```python
from build123d import *

# Parameters (mm, degrees)
SKETCH1_W           = 75
SKETCH1_H           = 75
SKETCH1_R           = 2.75
SKETCH1_R_2         = 16
BOSS_EXTRUDE1_DEPTH = 6
BOSS_EXTRUDE2_DEPTH = 75
SKETCH3_R           = 21.05
CUT_EXTRUDE1_DEPTH  = 6
SKETCH4_R           = 21.05
SKETCH4_R_2         = 19.05
BOSS_EXTRUDE3_DEPTH = 2
SKETCH5_R           = 3.25
CUT_EXTRUDE2_DEPTH  = 97.785892457
CUT_EXTRUDE3_DEPTH  = 6
SKETCH7_R           = 1.25
BOSS_EXTRUDE4_DEPTH = 10
SKETCH11_W          = 6.5
SKETCH11_H          = 26
CUT_EXTRUDE7_DEPTH  = 10


with BuildPart() as part:
    # Sketch1 → Boss-Extrude1 (new body)
    with BuildSketch(Plane.XY):
        Rectangle(SKETCH1_W, SKETCH1_H)
        with Locations((21, 21)):
            Circle(SKETCH1_R, mode=Mode.SUBTRACT)
        with Locations((21, -21)):
            Circle(SKETCH1_R, mode=Mode.SUBTRACT)
        with Locations((-21, -21)):
            Circle(SKETCH1_R, mode=Mode.SUBTRACT)
        with Locations((-21, 21)):
            Circle(SKETCH1_R, mode=Mode.SUBTRACT)
        Circle(SKETCH1_R_2, mode=Mode.SUBTRACT)
    extrude(amount=BOSS_EXTRUDE1_DEPTH)

    # Sketch2 → Boss-Extrude2 (add)
    with BuildSketch(Plane.ZY.offset(37.5)):
        Polygon((0, 37.5), (-50, 37.5), (-50, 69.464084092), (-55, 69.464084092), (-55, 32.5), (-36.09839393, 32.5), (-36.09839393, -32.5), (-55, -32.5), (-55, -69.464084092), (-50, -69.464084092), (-50, -37.5), (0, -37.5), (0, -32.5), (-30.09839393, -32.5), (-30.09839393, 32.5), (0, 32.5), align=None)
    extrude(amount=-BOSS_EXTRUDE2_DEPTH)

    # Sketch3 → Cut-Extrude1 (cut)
    with BuildSketch(Plane(origin=(0, 0, -36.09839393), x_dir=(-1, 0, 0), z_dir=(0, 0, -1))):
        Circle(SKETCH3_R)
    extrude(amount=-CUT_EXTRUDE1_DEPTH, mode=Mode.SUBTRACT)

    # Sketch4 → Boss-Extrude3 (add)
    with BuildSketch(Plane(origin=(0, 0, -36.09839393), x_dir=(-1, 0, 0), z_dir=(0, 0, -1))):
        Circle(SKETCH4_R)
        Circle(SKETCH4_R_2, mode=Mode.SUBTRACT)
    extrude(amount=-BOSS_EXTRUDE3_DEPTH)

    # Sketch5 → Cut-Extrude2 (cut, through all)
    with BuildSketch(Plane.XY.offset(-50)):
        with Locations((30, -60)):
            Circle(SKETCH5_R)
        with Locations((-30, -60)):
            Circle(SKETCH5_R)
    cut_extrude2 = extrude(amount=-CUT_EXTRUDE2_DEPTH, mode=Mode.SUBTRACT)

    # Mirror1: Cut-Extrude2 across plane
    add(cut_extrude2.mirror(Plane.ZX), mode=Mode.SUBTRACT)

    # Sketch6 → Cut-Extrude3 (cut)
    with BuildSketch(Plane(origin=(0, 0, -36.09839393), x_dir=(-1, 0, 0), z_dir=(0, 0, -1))):
        with BuildLine():
            Line((26, 23.5), (26, 18.5))
            ThreePointArc((26, 18.5), (21, 13.5), (16, 18.5))
            Line((16, 18.5), (16, 23.5))
            ThreePointArc((16, 23.5), (21, 28.5), (26, 23.5))
        make_face()
        with BuildLine():
            Line((16, -23.5), (16, -18.5))
            ThreePointArc((16, -18.5), (21, -13.5), (26, -18.5))
            Line((26, -18.5), (26, -23.5))
            ThreePointArc((26, -23.5), (21, -28.5), (16, -23.5))
        make_face()
        with BuildLine():
            Line((-16, -23.5), (-16, -18.5))
            ThreePointArc((-16, -18.5), (-21, -13.5), (-26, -18.5))
            Line((-26, -18.5), (-26, -23.5))
            ThreePointArc((-26, -23.5), (-21, -28.5), (-16, -23.5))
        make_face()
        with BuildLine():
            Line((-26, 23.5), (-26, 18.5))
            ThreePointArc((-26, 18.5), (-21, 13.5), (-16, 18.5))
            Line((-16, 18.5), (-16, 23.5))
            ThreePointArc((-16, 23.5), (-21, 28.5), (-26, 23.5))
        make_face()
    extrude(amount=-CUT_EXTRUDE3_DEPTH, mode=Mode.SUBTRACT)

    # Sketch7 → Boss-Extrude4 (add)
    # profile 1 of 2: a face of its own
    with BuildSketch(Plane(origin=(0, 0, -36.09839393), x_dir=(-1, 0, 0), z_dir=(0, 0, -1))):
        Polygon((-26, -3), (-21, -3), (-21, -13), (-37.5, -13), (-37.5, -10), (-26, -10), align=None)
        with Locations(Location((-23.5, -5, 0), (0, 0, 180))):
            Circle(SKETCH7_R, mode=Mode.SUBTRACT)
    # profile 2 of 2: a face of its own
    with BuildSketch(Plane(origin=(0, 0, -36.09839393), x_dir=(-1, 0, 0), z_dir=(0, 0, -1))):
        Polygon((-21, 13), (-37.5, 13), (-37.5, 10), (-26, 10), (-26, 3), (-21, 3), align=None)
        with Locations((-23.5, 5)):
            Circle(SKETCH7_R, mode=Mode.SUBTRACT)
    extrude(amount=BOSS_EXTRUDE4_DEPTH)

    # Sketch11 → Cut-Extrude7 (cut)
    with BuildSketch(Plane.ZY.offset(-21)):
        with Locations((-39.34839393, 0)):
            Rectangle(SKETCH11_W, SKETCH11_H)
    extrude(amount=-CUT_EXTRUDE7_DEPTH, mode=Mode.SUBTRACT)


solid = part.part
```
Geometry: final body of the model. Coordinates: model frame, mm. A direction names the side the tool comes from. Round coordinates to 2 decimals unless told otherwise and drop trailing zeros. Order: outer loops, then holes, each group sorted by start corner. A loop starts at its lowest first (then second) coordinate and runs counter-clockwise, first axis right, second up. Notation, with made-up numbers: (-28.75, 60.25) -> (8.25, 60.25) arc R27 ccw to (8.25, 86.25) -> close; hole circle Ø3 at (79, 3). An arc over 180 degrees is marked (long way). Write each question's results on one line, items separated by ' | '.
Q1. Pull-direction query (Y, two-part tool) for faces 1 (the face through (18.253, 21.121, 2.958)), 2 (the face through (-1, -37.5, -22)), 3 (the face through (-1, -54, -50)); classes: released by +Y, released by -Y, zero draft, split by the parting line, or undercut.
Response values:
face 1: undercut | face 2: released by -Y | face 3: zero draft
Q2. Section query C-C (y = 60). Output: boundary loops of the cut face in (x, z).
Response values:
outline: (-37.5, -55) -> (-33.25, -55) -> (-33.25, -50) -> (-37.5, -50) -> close; (-26.75, -55) -> (26.75, -55) -> (26.75, -50) -> (-26.75, -50) -> close; (33.25, -55) -> (37.5, -55) -> (37.5, -50) -> (33.25, -50) -> close
Q3. Section query D-D (y = -30.5). Output: boundary loops of the cut face in (x, z), and give its area (3 significant figures).
Response values:
outline: (-37.5, -36.1) -> (37.5, -36.1) -> (37.5, -30.1) -> (-37.5, -30.1) -> close; (-37.5, 0) -> (37.5, 0) -> (37.5, 6) -> (-37.5, 6) -> close | area: 900 mm²
Q4. Section query B-B (z = -40). Output: boundary loops of the cut face in (x, y), and give its area (3 significant figures).
Response values:
outline: (-37.5, -37.5) -> (37.5, -37.5) -> (37.5, -32.5) -> (-37.5, -32.5) -> close; (-37.5, 32.5) -> (37.5, 32.5) -> (37.5, 37.5) -> (-37.5, 37.5) -> close; (31, -13) -> (37.5, -13) -> (37.5, -10) -> (31, -10) -> close; (31, 10) -> (37.5, 10) -> (37.5, 13) -> (31, 13) -> close | area: 789 mm²
Q5. Access query for faces 4 (the face through (-1, 53, -50)), 5 (the face through (-21.1, -28.5, -33.1)), 6 (the face through (31, -11, -39)), 7 (the face through (24, -3, -44)). Directions: +Z, -Z, +X, -X, +Y, -Y. A direction counts if a zero-diameter tool reaches every point of the face in a straight line with its end or side. Return the directions, or none.
Response values:
face 4: +Z, +X, -X, +Y | face 5: -Z | face 6: -X | face 7: -Z, +X, -X
Q6. Pin query (flat end, axial travel): pin 1 Ø1.8 at (x, z) = (22.5, -45) entering from +Y; pin 2 Ø11 at (x, y) = (26, 9.5) entering from -Z; pin 3 Ø1.5 at (x, z) = (-0.5, -38.5) entering from -Y; pin 4 Ø5 at (x, y) = (21, 21) entering from -Z. Return the tip coordinate at first contact, or that it passes through.
Response values:
pin 1: y = 37.5 | pin 2: z = -46.1 | pin 3: y = -37.5 | pin 4: through
Q7. Ray query, line 1 along X through (y, z) = (60, -52.7); line 2 along Y through (x, z) = (30, -53); line 3 along Y through (x, z) = (-6.5, -13). Return the intervals inside material, ascending.
Response values:
line 1: -37.5 to -33.25, -26.75 to 26.75, 33.25 to 37.5 | line 2: -69.46 to -63.25, -56.75 to -32.5, 32.5 to 56.75, 63.25 to 69.46 | line 3: -37.5 to -32.5, 32.5 to 37.5
Q8. Section query A-A (x = -30). Output: boundary loops of the cut face in (y, z), and give its area (3 significant figures).
Response values:
outline: (-69.46, -55) -> (-63.25, -55) -> (-63.25, -50) -> (-69.46, -50) -> close; (-56.75, -55) -> (-32.5, -55) -> (-32.5, -36.1) -> (32.5, -36.1) -> (32.5, -55) -> (56.75, -55) -> (56.75, -50) -> (37.5, -50) -> (37.5, 6) -> (-37.5, 6) -> (-37.5, -50) -> (-56.75, -50) -> close; (63.25, -55) -> (69.46, -55) -> (69.46, -50) -> (63.25, -50) -> close; hole (-32.5, -30.1) -> (32.5, -30.1) -> (32.5, 0) -> (-32.5, 0) -> close | area: 1,640 mm²
